```python
from build123d import *

# Parameters (mm, degrees)
SKETCH2_R           = 2
BOSS_EXTRUDE1_DEPTH = 0.5
BOSS_EXTRUDE1_TAPER = -45
SKETCH3_R           = 2.5
BOSS_EXTRUDE2_DEPTH = 18.501
SKETCH4_R           = 1.15
BOSS_EXTRUDE3_DEPTH = 1.25
SKETCH5_R           = 1.15
BOSS_EXTRUDE4_DEPTH = 0.35
BOSS_EXTRUDE4_TAPER = -44.999999995
SKETCH6_R           = 1.5
BOSS_EXTRUDE5_DEPTH = 4.0935
SKETCH7_R           = 1.5
BOSS_EXTRUDE6_DEPTH = 0.3065
BOSS_EXTRUDE6_TAPER = 45
CUT_EXTRUDE1_DEPTH  = 1.6
CHAMFER1_SIZE       = 0.4


with BuildPart() as part:
    # Sketch1 → Revolve1 (revolve)
    with BuildSketch(Plane(origin=(0, 0, 0), x_dir=(-1, 0, 0), z_dir=(0, 0, -1))):
        with BuildLine():
            Line((-0.999, 2), (-0.999, 0))
            Line((-0.999, 0), (3.5, 0))
            Line((3.5, 0), (3.5, 4))
            Line((3.5, 4), (0, 4))
            Line((0, 4), (0, 2.75))
            ThreePointArc((0, 2.75), (-0.325180465, 2.142806379), (-0.999, 2))
        make_face()
    revolve(axis=Axis((0.999, 0, 0), (-1, 0, 0)))

    # Sketch2 → Boss-Extrude1 (add)
    with BuildSketch(Plane(origin=(0.999, 0, 0), x_dir=(0, 0, -1), z_dir=(1, 0, 0))):
        Circle(SKETCH2_R)
    extrude(amount=BOSS_EXTRUDE1_DEPTH, taper=BOSS_EXTRUDE1_TAPER)

    # Sketch3 → Boss-Extrude2 (add)
    with BuildSketch(Plane(origin=(1.499, 0, 0), x_dir=(0, 0, -1), z_dir=(1, 0, 0))):
        Circle(SKETCH3_R)
    extrude(amount=BOSS_EXTRUDE2_DEPTH)

    # Sketch4 → Boss-Extrude3 (add)
    with BuildSketch(Plane(origin=(20, 0, 0), x_dir=(0, 0, -1), z_dir=(1, 0, 0))):
        Circle(SKETCH4_R)
    extrude(amount=BOSS_EXTRUDE3_DEPTH)

    # Sketch5 → Boss-Extrude4 (add)
    with BuildSketch(Plane(origin=(21.25, 0, 0), x_dir=(0, 0, -1), z_dir=(1, 0, 0))):
        Circle(SKETCH5_R)
    extrude(amount=BOSS_EXTRUDE4_DEPTH, taper=BOSS_EXTRUDE4_TAPER)

    # Sketch6 → Boss-Extrude5 (add)
    with BuildSketch(Plane(origin=(21.6, 0, 0), x_dir=(0, 0, -1), z_dir=(1, 0, 0))):
        Circle(SKETCH6_R)
    extrude(amount=BOSS_EXTRUDE5_DEPTH)

    # Sketch7 → Boss-Extrude6 (add)
    with BuildSketch(Plane(origin=(25.6935, 0, 0), x_dir=(0, 0, -1), z_dir=(1, 0, 0))):
        Circle(SKETCH7_R)
    extrude(amount=BOSS_EXTRUDE6_DEPTH, taper=BOSS_EXTRUDE6_TAPER)

    # Sketch8 → Cut-Extrude1 (cut)
    with BuildSketch(Plane.ZY.offset(3.5)):
        Polygon((0, 1.443375673), (-1.25, 0.721687836), (-1.25, -0.721687836), (0, -1.443375673), (1.25, -0.721687836), (1.25, 0.721687836), align=None)
    extrude(amount=-CUT_EXTRUDE1_DEPTH, mode=Mode.SUBTRACT)

    # Sketch9 → Cut-Revolve1 (revolve, cut)
    with BuildSketch(Plane.XY):
        Polygon((-1.9, 1.25), (-1.9, 0), (-1.178312164, 0), align=None)
    revolve(axis=Axis((-1.9, 0, 0), (1, 0, 0)), mode=Mode.SUBTRACT)

    # Chamfer1
    chamfer1_edges = [part.edges().sort_by_distance(p)[0] for p in [
        (-3.5, -4, 0),
    ]]
    chamfer(chamfer1_edges, length=CHAMFER1_SIZE)


solid = part.part
```
Build history of the part. All positions in model axes, mm. A direction names the side the tool comes from. Round coordinates to 2 decimals unless told otherwise and drop trailing zeros. Write each loop counter-clockwise with the first axis right and the second up, starting at its lowest first coordinate (ties: lowest second). Pieces come first, ordered by that corner, then holes.
1) 3-axis set-ups, long thin cutter, end or side, ignore diameter. For faces 4 (the cylindrical face through (23.62, 0.07, 1.5)), 5 (the flat face through (-2.71, -1.08, -0.63)), 6 (the cylindrical face through (-1.528, -0.867, 3.905)): which of +Z, -Z, +X, -X, +Y, -Y reach the whole face in a straight line?
2) Mould opens along X. For faces 1 (the flat face through (-3.5, 0, 2)), 2 (the flat face through (20, -1, -1)), 3 (the flat face through (-3, 0, -1.25)) say: +X half, -X half, draft (parallel to the pull), parting line (faces both ways), or undercut.
3) Band-saw the part on B-B, the plane x = 23. List the corners of the cut face in (y, z).
4) Drill centre lines: probe 1 along X at (y, z) = (2.25, 1.75); probe 2 along X at (y, z) = (-1.5, -1.25); probe 3 along Z at (x, y) = (-0.75, 1.75). Where is each one in solid material? Low to high.
5) Band-saw the part on A-A, the plane x = -0.75. List the corners of the cut face in (y, z), and give its area (3 significant figures).
6) Pin check, flat tips, straight feed: pin 1 (1.5 mm diameter, centred on x = 4, z = -1.5, fed in from -Y); pin 2 (1.5 mm diameter, centred on x = 15, y = -1, fed in from +Z); pin 3 (2 mm diameter, centred on x = 10.5, y = -2.5, fed in from +Z). Stop position of each tip, or through.
Ans:
1. face 4: +X
1. face 5: -X
1. face 6: +X, -X
2. face 1: -X half
2. face 2: undercut
2. face 3: draft
3. outline: circle Ø3 at (0, 0)
4. probe 1: x = -3.5 to 0
4. probe 2: x = -3.5 to 20
4. probe 3: z = -3.6 to 3.6
5. outline: circle Ø8 at (0, 0)
5. area: 50.3 mm2
6. pin 1: stops at y = -2.38
6. pin 2: stops at z = 2.49
6. pin 3: stops at z = 2
